Verification items for the finished model (mm, model axes). Face numbers are marked on the shaded views. A direction names the side the tool comes from. Round coordinates to 2 decimals unless told otherwise and drop trailing zeros. Order: outer loops, then holes, each group sorted by start corner. A loop starts at its lowest first (then second) coordinate and runs counter-clockwise, first axis right, second up. Notation, with made-up numbers: M 33,-35.5 L 80,-35.5 A24 ccw 80,-25.5 Z; hole C 39.25,22.25 d4. An arc over 180 degrees is marked long. Use one line per item in the form item = value. Start each with the question number.
Item 1: Cross-section at C-C on x = -7.5. Enter the section's corners in (y, z).
Item 2: Tool access check on the marked faces 1 and 2. Record the directions out of +Z, -Z, +X, -X, +Y, -Y that give a thin tool (end or side, any length) a straight path to the whole face; none if there is none.
Item 3: Thickness scan on probe 1 along Z at (x, y) = (-0.55, 15); probe 2 along X at (y, z) = (0.75, 12.5); probe 3 along Y at (x, z) = (-5, 19). Record the ranges inside material, lowest first. Write a range as [from, to].
Item 4: Cross-section at D-D on x = -9.5. Enter the section's corners in (y, z), then the cut area to 3 significant figures.
Item 5: Go/stop test with flat-tipped pins: pin 1 Ø3 at (x, z) = (-3.5, 17.5) entering from -Y; pin 2 Ø1.9 at (y, z) = (15, 15.25) entering from -X; pin 3 Ø4 at (x, z) = (-5, 3) entering from +Y. Record where each tip stops, or that it passes through.
Item 6: Cross-section at A-A on z = 15.25. Enter the section's corners in (x, y).
Item 7: Cross-section at B-B on y = 15. Enter the section's corners in (x, z), then the cut area to 3 significant figures.
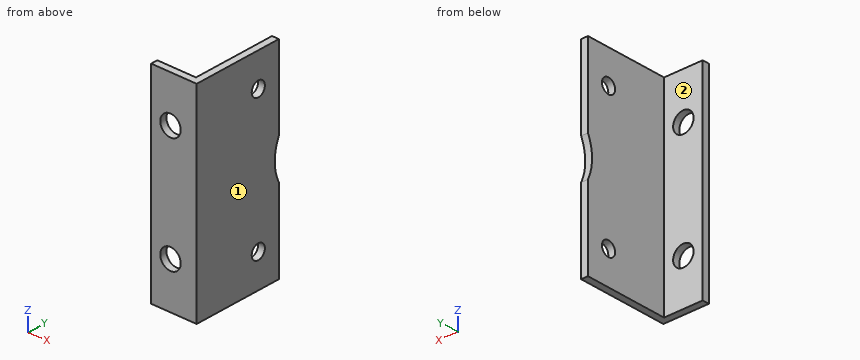
Autodesk Inventor part; units mm, degrees
ref_plane "YZ Plane" through (0, 0, 0) normal (1, 0, 0) x (0, 1, 0)
ref_plane "XZ Plane" through (0, 0, 0) normal (0, 1, 0) x (-1, 0, 0)
ref_plane "XY Plane" through (0, 0, 0) normal (0, 0, 1) x (1, 0, 0)
sketch "Náčrt1" plane through (0, 0, 0) normal (0, 0, 1) x (1, 0, 0)
  line L0 (-10, 0) -> (0, 0)
  line L1 (0, 0) -> (0, 20)
  line L2 (0, 20) -> (-1.5, 20)
  line L3 (-1.5, 20) -> (-1.5, 1.5)
  line L4 (-1.5, 1.5) -> (-10, 1.5)
  line L5 (-10, 1.5) -> (-10, 0)
  line L6 (-12, 0) -> (2, 0)
  line L7 (0, 24) -> (0, -4)
  point P0 (0, 0)
  dimension "d0" = 20
  dimension "d1" = 10
  dimension "d2" = 1.5
  dimension "d3" = 1.5
extrude "Vysunutí1" add sketch "Náčrt1" along normal mid plane 45
sketch "Náčrt2" plane through (-10, 1.5, 22.5) normal (0, 1, 0) x (1, 0, 0)
  line L0 (0, 0) -> (0, 45)
  line L1 (8.5, 0) -> (0, 0)
  line L2 (8.5, 45) -> (8.5, 0)
  line L3 (0, 45) -> (8.5, 45)
  point P0 (10, 22.5)
  point P1 (4.25, 35)
  point P2 (4.25, 10)
  point P3 (4.25, 0)
  dimension "d6" = 4.25
  dimension "d7" = 4.25
  dimension "d8" = 25
  dimension "d9" = 10
hole "Díra1" at (-5.75, 1.5, -12.5) at (-5.75, 1.5, 12.5) direction (0, -1, 0) diameter 4.5 end through all
sketch "Náčrt5" plane through (0, 0, 22.5) normal (1, 0, 0) x (0, 0, -1)
  line L0 (45, 20) -> (0, 20)
  line L1 (0, 0) -> (0, 20)
  line L2 (45, 0) -> (0, 0)
  line L3 (45, 20) -> (45, 0)
  line L4 (22.5, 0) -> (22.5, 47.1534) construction
  point P0 (22.5, 20)
  point P1 (37.75, 15)
  point P2 (7.25, 15)
  dimension "d41" = 30.5
  dimension "d42" = 5
  dimension "d43" = 47.1534
hole "Díra4" at (0, 15, -15.25) at (0, 15, 15.25) direction (-1, 0, 0) diameter 3.2 end through all
sketch "Náčrt6" plane through (0, 0, 22.5) normal (1, 0, 0) x (0, 0, -1)
  line L0 (22.5, 0) -> (22.5, 40) construction
  circle A0 centre (22.5, 29) radius 10
  point P0 (22.5, 19)
  point P1 (22.5, 20)
  dimension "d52" = 20
  dimension "d51" = 40
  dimension "d53" = 1
extrude "Vysunutí2" cut sketch "Náčrt6" against normal through all
properties part number "x_bracket_stepper" material "Hliník 6061"
Output values:
q1.outline = M 0,-22.5 L 1.5,-22.5 L 1.5,-13.91 L 0,-13.91 Z; M 0,-11.09 L 1.5,-11.09 L 1.5,11.09 L 0,11.09 Z; M 0,13.91 L 1.5,13.91 L 1.5,22.5 L 0,22.5 Z
q2.face_1 = +Z, -Z, +X, +Y, -Y
q2.face_2 = +Z, -Z, -X, +Y
q3.probe_1 = [-22.5, -16.85], [-13.65, 13.65], [16.85, 22.5]
q3.probe_2 = [-10, -8], [-3.5, 0]
q3.probe_3 = [0, 1.5]
q4.outline = M 0,-22.5 L 1.5,-22.5 L 1.5,22.5 L 0,22.5 Z
q4.area = 67.5 mm2
q5.pin_1 = 0
q5.pin_2 = through
q5.pin_3 = 1.5
q6.outline = M -10,0 L 0,0 L 0,13.4 L -1.5,13.4 L -1.5,1.5 L -10,1.5 Z; M -1.5,16.6 L 0,16.6 L 0,20 L -1.5,20 Z
q7.outline = M -1.5,-22.5 L 0,-22.5 L 0,-16.85 L -1.5,-16.85 Z; M -1.5,-13.65 L 0,-13.65 L 0,13.65 L -1.5,13.65 Z; M -1.5,16.85 L 0,16.85 L 0,22.5 L -1.5,22.5 Z
q7.area = 57.9 mm2
